```python
from build123d import *

# Parameters (mm, degrees)
SKETCH_W        = 60
SKETCH_H        = 25
PAD_DEPTH       = 6
SKETCH001_W     = 65
SKETCH001_H     = 8.25
POCKET_DEPTH    = 1
SKETCH002_W     = 6
SKETCH002_H     = 7.5
POCKET001_DEPTH = 10
CHAMFER_SIZE    = 4.5
SKETCH006_R     = 1.25
HOLE001_DEPTH   = 15
CHAMFER002_SIZE = 2
POCKET006_DEPTH = 10


with BuildPart() as part:
    # Sketch → Pad (new body)
    with BuildSketch(Plane.XY):
        Rectangle(SKETCH_W, SKETCH_H)
    extrude(amount=PAD_DEPTH)

    # Sketch001 → Pocket (cut)
    with BuildSketch(Plane.XY.offset(5.5)):
        with Locations((0, 1.125)):
            Rectangle(SKETCH001_W, SKETCH001_H)
    extrude(amount=POCKET_DEPTH, mode=Mode.SUBTRACT)

    # Sketch002 → Pocket001 (cut)
    with BuildSketch(Plane.XY):
        with Locations((0, 1)):
            Rectangle(SKETCH002_W, SKETCH002_H)
    extrude(amount=POCKET001_DEPTH, mode=Mode.SUBTRACT)

    # Chamfer
    chamfer_edges = [part.edges().sort_by_distance(p)[0] for p in [
        (0, 4.75, 0),
        (-3, 1, 0),
        (0, -2.75, 0),
        (3, 1, 0),
        (-30, 1.125, 5.5),
        (30, 1.125, 5.5),
    ]]
    chamfer(chamfer_edges, length=CHAMFER_SIZE)

    # Sketch006 → Hole001 (cut)
    with BuildSketch(Plane.XY):
        with Locations((-15, 7.5)):
            Circle(SKETCH006_R)
        with Locations((15, 7.5)):
            Circle(SKETCH006_R)
        with Locations((-10, -7.5)):
            Circle(SKETCH006_R)
        with Locations((10, -7.5)):
            Circle(SKETCH006_R)
    extrude(amount=HOLE001_DEPTH, mode=Mode.SUBTRACT)

    # Chamfer002
    chamfer002_edges = [part.edges().sort_by_distance(p)[0] for p in [
        (-30, -12.5, 3),
        (-30, 12.5, 3),
        (30, -12.5, 3),
        (30, 12.5, 3),
    ]]
    chamfer(chamfer002_edges, length=CHAMFER002_SIZE)

    # Sketch015 → Pocket006 (cut)
    with BuildSketch(Plane.XY):
        with BuildLine():
            ThreePointArc((-25, -5.85), (-26.65, -7.5), (-25, -9.15))
            Line((-25, -9.15), (-17, -9.15))
            ThreePointArc((-17, -9.15), (-15.35, -7.5), (-17, -5.85))
            Line((-25, -5.85), (-17, -5.85))
        make_face()
        with BuildLine():
            ThreePointArc((17, -5.85), (15.35, -7.5), (17, -9.15))
            Line((17, -9.15), (25, -9.15))
            ThreePointArc((25, -9.15), (26.65, -7.5), (25, -5.85))
            Line((17, -5.85), (25, -5.85))
        make_face()
    extrude(amount=POCKET006_DEPTH, mode=Mode.SUBTRACT)


solid = part.part
```
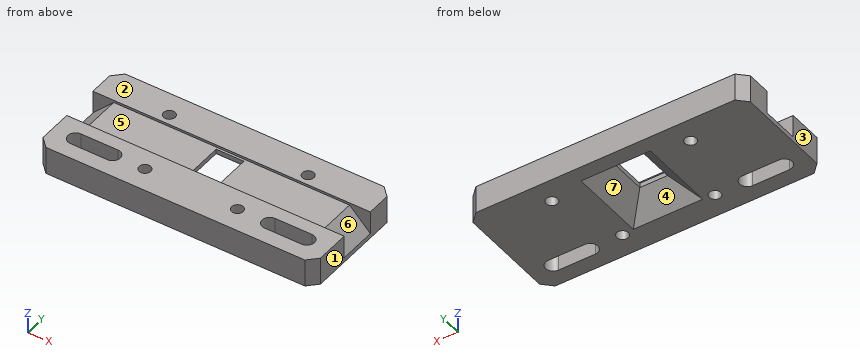
The listing builds one solid part. Answer for the finished solid, in the listing's coordinates (mm). Face numbers are marked on the shaded views. A direction names the side the tool comes from. Give positions to 0.01 mm unless a question says otherwise; leave off trailing zeros. Order: outer loops, then holes, each group sorted by start corner. A loop starts at its lowest first (then second) coordinate and runs counter-clockwise, first axis right, second up. Notation, with made-up numbers: (84.25, 59) -> (128.25, 59) arc R24 cw to (128.25, 78) -> close; hole circle Ø4 at (-33.5, 21.5). An arc over 180 degrees is marked (long way). Answer as a JSON object with one key per item and string values. Group by question number.
Item 1: Flat-ended cylindrical pins translate along their axes: pin 1 (0.5 mm diameter, centred on y = 2, z = 5, fed in from -X); pin 2 (0.5 mm diameter, centred on y = 0.5, z = 5, fed in from +X). Find the tip coordinate at first contact, or state that the pin passes through.
Item 2: A tool of negligible diameter and unlimited length cuts with its end or side. For the marked faces 5, 6 and 7, from which of +Z, -Z, +X, -X, +Y, -Y can it reach the whole face along a straight path? Write none if from no direction.
Item 3: Consider L1, parallel to X at y = 7.5, z = 1.8; L2, parallel to X at y = -7.5, z = 1.6; L3, parallel to Y at x = -27, z = 4.5. Determine where each line is inside the solid, lowest interval first. Write a range as from..to.
Item 4: The part is cut by section D-D on z = 2. Give the number of separate pieces and of enclosed holes in the cut face, and give its area (3 significant figures).
Item 5: The part is cut by section B-B on y = 0.5. Write down the section's boundary in (x, z), and give its area (4 significant figures).
Item 6: Determine the mould class of the marked faces 1, 2, 3 and 4 for opening direction X: pulls with the +X half, pulls with the -X half, needs draft (parallel to the pull), parting line crosses it, or undercut.
Item 7: The part is cut by section C-C on y = -4.75. Write down the section's boundary in (x, z), and give its area (3 significant figures).
Item 8: The part is cut by section A-A on x = 10. Write down the section's boundary in (y, z), and give its area (3 significant figures).
Result set:
{
 "1": {"pin 1": "x = -26.25", "pin 2": "x = 26.25"},
 "2": {"face 5": "+Z, +X, -X", "face 6": "+Z, +X", "face 7": "-Z"},
 "3": {"L1": "-30..-16.25, -13.75..13.75, 16.25..30", "L2": "-30..-26.65, -15.35..-11.25, -8.75..8.75, 11.25..15.35, 26.65..30", "L3": "-12.5..-3, 5.25..12.5"},
 "4": {"separate pieces": "1", "enclosed holes": "7", "area": "1,250 mm²"},
 "5": {"outline": "(-30, 0) -> (-7.5, 0) -> (-3, 4.5) -> (-3, 5.5) -> (-25.5, 5.5) -> (-30, 1) -> close; (3, 4.5) -> (7.5, 0) -> (30, 0) -> (30, 1) -> (25.5, 5.5) -> (3, 5.5) -> close", "area": "256.5 mm²"},
 "6": {"face 1": "pulls with the +X half", "face 2": "needs draft", "face 3": "pulls with the -X half", "face 4": "undercut"},
 "7": {"outline": "(-30, 0) -> (-7.5, 0) -> (-5, 2.5) -> (5, 2.5) -> (7.5, 0) -> (30, 0) -> (30, 6) -> (-30, 6) -> close", "area": "329 mm²"},
 "8": {"outline": "(-12.5, 0) -> (-8.75, 0) -> (-8.75, 6) -> (-12.5, 6) -> close; (-6.25, 0) -> (12.5, 0) -> (12.5, 6) -> (5.25, 6) -> (5.25, 5.5) -> (-3, 5.5) -> (-3, 6) -> (-6.25, 6) -> close", "area": "131 mm²"}
}
